For this review, take the finished solid that the model builds, in its own axes (mm). Face numbers are marked on the shaded views. A direction names the side the tool comes from. Round coordinates to 2 decimals unless told otherwise and drop trailing zeros. Order: outer loops, then holes, each group sorted by start corner. A loop starts at its lowest first (then second) coordinate and runs counter-clockwise, first axis right, second up. Notation, with made-up numbers: M 46.25,86.25 L 58.25,86.25 A15 ccw 58.25,107.25 Z; hole C 55,67.5 d8. An arc over 180 degrees is marked long. Put each result on its own line as item: value.
from build123d import *

# Parameters (mm, degrees)
F0_W     = 15.8242
F0_H     = 7.9121
F2_DEPTH = 9.6012
F1_R     = 2.4511
F3_DEPTH = 1.778
F4_W     = 13.335
F4_H     = 5.4229
F6_DEPTH = 7.62
F5_R     = 1.478616
F7_DEPTH = 8.128


with BuildPart() as f2:
    # F0 (on Top) → F2 (new body)
    with BuildSketch(Plane.XY):
        Rectangle(F0_W, F0_H)
    extrude(amount=F2_DEPTH)

    # F1 (on face) → F3 (join)
    with BuildSketch(Plane.XY):
        with Locations((-3.9624, 0)):
            Circle(F1_R)
        with Locations((3.9624, 0)):
            Circle(F1_R)
    extrude(amount=-F3_DEPTH)

    # F4 (on face) → F6 (cut)
    with BuildSketch(Plane.XY.offset(9.6012)):
        Rectangle(F4_W, F4_H)
    extrude(amount=-F6_DEPTH, mode=Mode.SUBTRACT)

    # F5 (on face) → F7 (join)
    with BuildSketch(Plane.XY.offset(9.6012)):
        Circle(F5_R)
    extrude(amount=-F7_DEPTH)


solid = f2.part
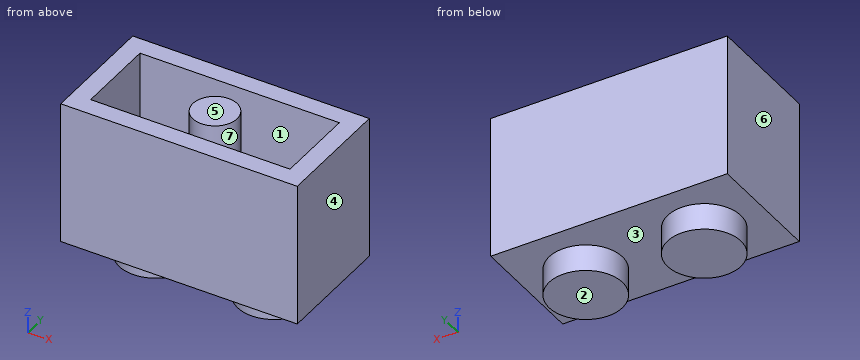
(1) For the marked faces 1, 2 and 3, list the 3-axis set-ups (+Z, -Z, +X, -X, +Y, -Y) from which the entire face can be reached by the end or side of a thin tool; tool diameter is ignored.
A:
face 1: +Z
face 2: -Z, +X, -X, +Y, -Y
face 3: -Z
(2) Add section B-B on x = 0. Give the boundary of the cut face in (y, z).
A:
outline: M -3.96,0 L 3.96,0 L 3.96,9.6 L 2.71,9.6 L 2.71,1.98 L 1.48,1.98 L 1.48,9.6 L -1.48,9.6 L -1.48,1.98 L -2.71,1.98 L -2.71,9.6 L -3.96,9.6 Z
(3) Add section A-A on z = 7.5. Give the boundary of the cut face in (x, y).
A:
outline: M -7.91,-3.96 L 7.91,-3.96 L 7.91,3.96 L -7.91,3.96 Z; C 0,0 d2.96; hole M -6.67,-2.71 L 6.67,-2.71 L 6.67,2.71 L -6.67,2.71 Z
(4) Insertion check: pin 1 Ø2.5 at (x, y) = (3, 0) entering from +Z. The pin has a flat end and moves straight along its axis. Give the tip position at first contact, or say it passes through.
A:
pin 1: stops at z = 1.98
(5) Draft analysis for pull direction X (two halves, no side actions). For the marked faces 4, 5, 6 and 7, state which applies: released by +X, released by -X, zero draft, split by the parting line, or undercut.
A:
face 4: released by +X
face 5: zero draft
face 6: released by -X
face 7: undercut
(6) Add section C-C on y = -0.5. Give the boundary of the cut face in (x, z), then the cut area to 3 significant figures.
A:
outline: M -7.91,0 L -6.36,0 L -6.36,-1.78 L -1.56,-1.78 L -1.56,0 L 1.56,0 L 1.56,-1.78 L 6.36,-1.78 L 6.36,0 L 7.91,0 L 7.91,9.6 L 6.67,9.6 L 6.67,1.98 L 1.39,1.98 L 1.39,9.6 L -1.39,9.6 L -1.39,1.98 L -6.67,1.98 L -6.67,9.6 L -7.91,9.6 Z
area: 88.6 mm2
(7) Add section D-D on y = 1. Give the boundary of the cut face in (x, z), then the cut area to 3 significant figures.
A:
outline: M -7.91,0 L -6.2,0 L -6.2,-1.78 L -1.72,-1.78 L -1.72,0 L 1.72,0 L 1.72,-1.78 L 6.2,-1.78 L 6.2,0 L 7.91,0 L 7.91,9.6 L 6.67,9.6 L 6.67,1.98 L 1.09,1.98 L 1.09,9.6 L -1.09,9.6 L -1.09,1.98 L -6.67,1.98 L -6.67,9.6 L -7.91,9.6 Z
area: 82.8 mm2
(8) To check wall thickness, follow L1, parallel to Y at x = 0, z = 6; L2, parallel to X at y = -1.25, z = 4; L3, parallel to X at y = 2.5, z = 6. State the ranges of each line that lie inside material, in increasing order.
A:
L1: y = -3.96 to -2.71, -1.48 to 1.48, 2.71 to 3.96
L2: x = -7.91 to -6.67, -0.79 to 0.79, 6.67 to 7.91
L3: x = -7.91 to -6.67, 6.67 to 7.91
